Geometry: final body of the model. Coordinates: model frame, mm. A direction names the side the tool comes from. Give positions to 0.01 mm unless a question says otherwise; leave off trailing zeros. Loops run counter-clockwise (first coordinate to the right, second up) from the corner with the lowest first, then second, coordinate; pieces in that order, holes last. Notation, with made-up numbers: (74, -7.5) -> (115, -7.5) arc R31 cw to (115, 22.5) -> close; hole circle Ø7 at (-22.75, 81). An arc over 180 degrees is marked (long way). Answer in a Markdown table with one row per item. Add a question column.
from build123d import *

# Parameters (mm, degrees)
F0_W     = 88.9
F0_H     = 88.9
F0_H_2   = 317.5
F1_DEPTH = 19.05
F0_W_2   = 438.15
F0_W_3   = 19.05
F2_DEPTH = 19.05


with BuildPart() as f1:
    # F0 (on Front) → F1 (new body)
    with BuildSketch(Plane.XZ):
        with Locations((-527.05, 0)):
            Rectangle(F0_W, F0_H)
        with Locations((-527.05, 203.2)):
            Rectangle(F0_W, F0_H_2)
    extrude(amount=-F1_DEPTH)



with BuildPart() as f1b:
    # F0 (on Front) → F1, piece 2 (new body)
    with BuildSketch(Plane.XZ):
        Rectangle(F0_W, F0_H)
        with Locations((0, 203.2)):
            Rectangle(F0_W, F0_H_2)
    extrude(amount=-F1_DEPTH)


with BuildPart() as f1c:
    # F0 (on Front) → F1, piece 3 (new body)
    with BuildSketch(Plane.XZ):
        with Locations((527.05, 0)):
            Rectangle(F0_W, F0_H)
        with Locations((527.05, 203.2)):
            Rectangle(F0_W, F0_H_2)
    extrude(amount=-F1_DEPTH)


with BuildPart() as f1_1:
    add(f1.part)

    add(f1b.part)  # F2 merges F1b

    add(f1c.part)  # F2 merges F1c
    # F0 (on Front) → F2 (join)
    with BuildSketch(Plane.XZ):
        with Locations((-263.525, 0)):
            Rectangle(F0_W_2, F0_H)
        with Locations((-527.05, 0)):
            Rectangle(F0_W, F0_H)
        with Locations((-581.025, 0)):
            Rectangle(F0_W_3, F0_H)
        Rectangle(F0_W, F0_H)
        with Locations((263.525, 0)):
            Rectangle(F0_W_2, F0_H)
        with Locations((527.05, 0)):
            Rectangle(F0_W, F0_H)
        with Locations((581.025, 0)):
            Rectangle(F0_W_3, F0_H)
    extrude(amount=F2_DEPTH)


solid = f1_1.part
(1) Material intervals for line 1 along X through (y, z) = (14.5, 301.5); line 2 along Z through (x, y) = (393, -6); line 3 along Y through (x, z) = (96.5, -11), sorted ascending. Write a range as from..to.
(2) Cut plane A-A on z = 235. Return the cut outline in (x, y).
(3) Draft query along X for faces 1 (the flat face through (-581, 0, 1)), 2 (the flat face through (-267, 0, 1)), 3 (the flat face through (-571.5, 9, 162)). Return one class per face: +X half, -X half, draft (parallel to the pull), parting line (faces both ways), or undercut.
(4) Pin query (flat end, axial travel): pin 1 Ø2 at (y, z) = (0, 49) entering from -X; pin 2 Ø21 at (x, z) = (582.5, -14) entering from +Y; pin 3 Ø21 at (y, z) = (12, 65) entering from +X. Return the tip coordinate at first contact, or that it passes through.
(5) Cut plane C-C on x = -245. Return the cut outline in (y, z).
(6) Cut plane B-B on y = 10. Return the cut outline in (x, z).
(7) Reachability of faces 4 (the flat face through (571.5, 9, 156)), 5 (the flat face through (482.6, 9, 162)), 6 (the flat face through (8, -9, 44.45)) from +Z, -Z, +X, -X, +Y, -Y: full face, straight path, thin tool, end or side. Return the list, or none.
Answer list:
| question | item | result |
|---|---|---|
| 1 | line 1 | x = -571.5..-482.6, -44.45..44.45, 482.6..571.5 |
| 1 | line 2 | z = -44.45..44.45 |
| 1 | line 3 | y = -19.05..0 |
| 2 | outline | (-571.5, 0) -> (-482.6, 0) -> (-482.6, 19.05) -> (-571.5, 19.05) -> close; (-44.45, 0) -> (44.45, 0) -> (44.45, 19.05) -> (-44.45, 19.05) -> close; (482.6, 0) -> (571.5, 0) -> (571.5, 19.05) -> (482.6, 19.05) -> close |
| 3 | face 1 | draft |
| 3 | face 2 | undercut |
| 3 | face 3 | -X half |
| 4 | pin 1 | stops at x = -571.5 |
| 4 | pin 2 | stops at y = 0 |
| 4 | pin 3 | stops at x = 571.5 |
| 5 | outline | (-19.05, -44.45) -> (0, -44.45) -> (0, 44.45) -> (-19.05, 44.45) -> close |
| 6 | outline | (-571.5, -44.45) -> (-482.6, -44.45) -> (-482.6, 361.95) -> (-571.5, 361.95) -> close; (-44.45, -44.45) -> (44.45, -44.45) -> (44.45, 361.95) -> (-44.45, 361.95) -> close; (482.6, -44.45) -> (571.5, -44.45) -> (571.5, 361.95) -> (482.6, 361.95) -> close |
| 7 | face 4 | +Z, -Z, +X, +Y |
| 7 | face 5 | +Z, -Z, +Y |
| 7 | face 6 | +Z, +X, -X, -Y |
